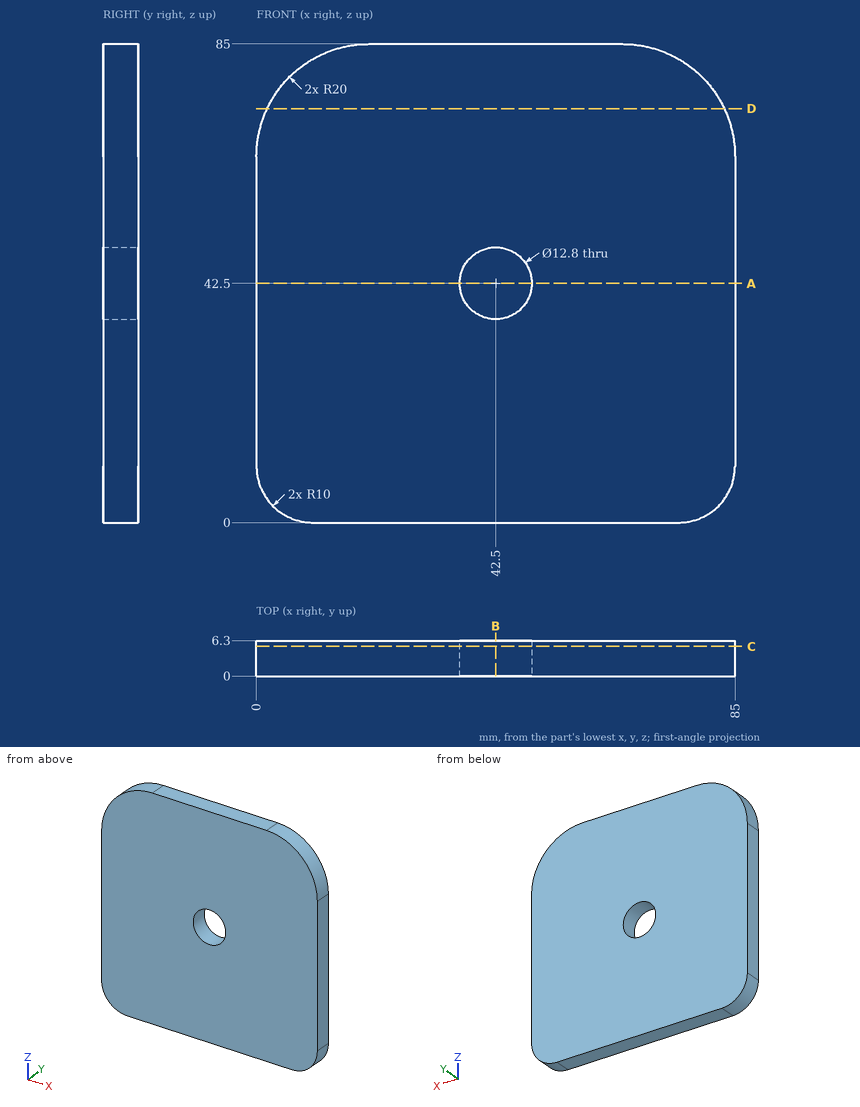
Input: dimensioned drawing with shaded views. Units: mm. Origin: part minimum x, y, z. Round coordinates to 2 decimals unless told otherwise and drop trailing zeros. Loops run counter-clockwise (first coordinate to the right, second up) from the corner with the lowest first, then second, coordinate; pieces in that order, holes last. Notation, with made-up numbers: (31.5, 77.25) -> (76.5, 77.25) arc R14 cw to (76.5, 87.25) -> close; hole circle Ø10 at (-1, 83). An arc over 180 degrees is marked (long way). Use one line per item in the form item = value. Start each with the question number.
1) Line query: L1, parallel to Z at x = 42.5, y = 3; L2, parallel to Z at x = 44, y = 2.25. Output: solid intervals per line, ascending.
2) Section B-B on x = 42.5. Output: boundary loops of the cut face in (y, z), then the cut area to 3 significant figures.
3) Section D-D on z = 73.5. Output: boundary loops of the cut face in (x, y), then the cut area to 3 significant figures.
4) Section A-A on z = 42.5. Output: boundary loops of the cut face in (x, y), then the cut area to 3 significant figures.
5) First-contact query: P1, Ø1, axis at y = 5.5, z = 74, coming from the +X side. Flat tip, straight axial feed; report the tip coordinate or a pass-through.
6) Section C-C on y = 5.25. Output: boundary loops of the cut face in (x, z), then the cut area to 3 significant figures.
Response:
q1.L1 = 0 to 36.1, 48.9 to 85
q1.L2 = 0 to 36.28, 48.72 to 85
q2.outline = (0, 0) -> (6.3, 0) -> (6.3, 36.1) -> (0, 36.1) -> close; (0, 48.9) -> (6.3, 48.9) -> (6.3, 85) -> (0, 85) -> close
q2.area = 455 mm^2
q3.outline = (1.9, 0) -> (83.1, 0) -> (83.1, 6.3) -> (1.9, 6.3) -> close
q3.area = 512 mm^2
q4.outline = (0, 0) -> (36.1, 0) -> (36.1, 6.3) -> (0, 6.3) -> close; (48.9, 0) -> (85, 0) -> (85, 6.3) -> (48.9, 6.3) -> close
q4.area = 455 mm^2
q5.P1 = 83.1
q6.outline = (0, 10) arc R10 ccw to (10, 0) -> (75, 0) arc R10 ccw to (85, 10) -> (85, 65) arc R20 ccw to (65, 85) -> (20, 85) arc R20 ccw to (0, 65) -> close; hole circle Ø12.8 at (42.5, 42.5)
q6.area = 6,880 mm^2
